Job drawing, mm, ordinate dimensions from the low corner. One solid piece. Round coordinates to 2 decimals unless told otherwise and drop trailing zeros. Loops run counter-clockwise (first coordinate to the right, second up) from the corner with the lowest first, then second, coordinate; pieces in that order, holes last.
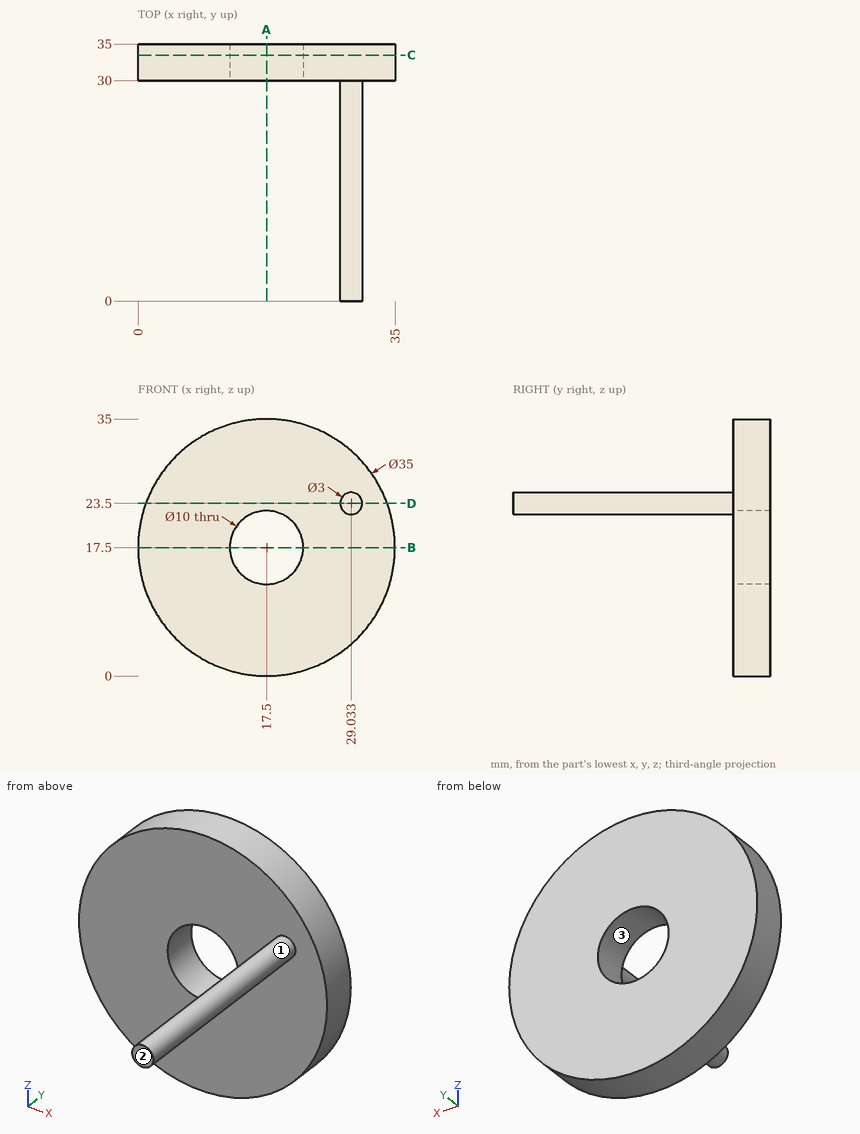
1) Slice it at A-A, the plane x = 17.5. Give the cut face in (y, z).
Values:
outline: (30, 0) - (35, 0) - (35, 12.5) - (30, 12.5) - close; (30, 22.5) - (35, 22.5) - (35, 35) - (30, 35) - close
2) Wall check: line 1 along Z through (x, y) = (17.5, 32.85); line 2 along Y through (x, z) = (4, 25); line 3 along Z through (x, y) = (33, 31) (1 decimal). Give the ranges that are in metal, low to high.
Values:
line 1: z = 0 to 12.5, 22.5 to 35
line 2: y = 30 to 35
line 3: z = 9.4 to 25.6
3) Slice it at C-C, the plane y = 33.5. Give the cut face in (x, z).
Values:
outline: circle Ø35 at (17.5, 17.5); hole circle Ø10 at (17.5, 17.5)
4) Mould opens along Z. For the marked faces 1, 2 and 3 say: released by +Z, released by -Z, zero draft, split by the parting line, or undercut.
Values:
face 1: split by the parting line
face 2: zero draft
face 3: undercut
5) Drop flat-ended pins along their axis: pin 1 Ø5 at (x, y) = (27.5, 20) entering from +Z; pin 2 Ø1 at (x, z) = (4.5, 28.5) entering from -Y; pin 3 Ø5 at (x, y) = (28, 22) entering from -Z; pin 4 Ø8 at (y, z) = (31.5, 13.5) entering from +X. Give the stop position or say it passes through.
Values:
pin 1: stops at z = 25
pin 2: stops at y = 30
pin 3: stops at z = 22
pin 4: stops at x = 35
6) Slice it at D-D, the plane z = 23.5. Give the cut face in (x, y).
Values:
outline: (1.06, 30) - (27.53, 30) - (27.53, 0) - (30.53, 0) - (30.53, 30) - (33.94, 30) - (33.94, 35) - (1.06, 35) - close
7) Slice it at B-B, the plane z = 17.5. Give the cut face in (x, y), then the cut area to 3 significant figures.
Values:
outline: (0, 30) - (12.5, 30) - (12.5, 35) - (0, 35) - close; (22.5, 30) - (35, 30) - (35, 35) - (22.5, 35) - close
area: 125 mm2
